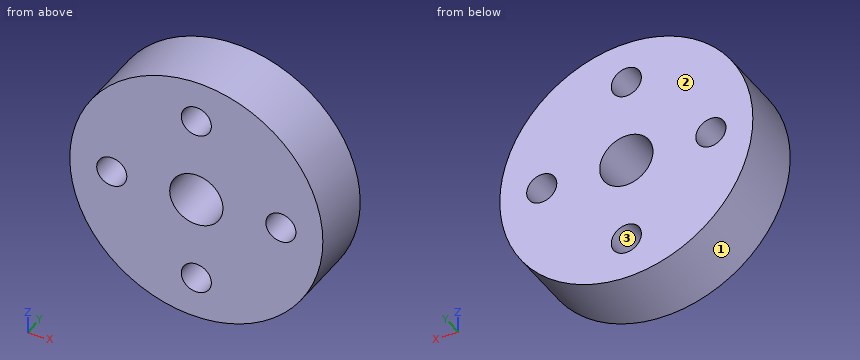
Autodesk Inventor part; units mm, degrees
ref_plane "YZ Plane" through (0, 0, 0) normal (1, 0, 0) x (0, 1, 0)
ref_plane "XZ Plane" through (0, 0, 0) normal (0, 1, 0) x (-1, 0, 0)
ref_plane "XY Plane" through (0, 0, 0) normal (0, 0, 1) x (1, 0, 0)
sketch "Sketch1" plane through (0, 0, 0) normal (0, 1, 0) x (-1, 0, 0)
  circle A0 centre (0, 0) radius 9.5
  circle A1 centre (0, 0) radius 2
  circle A2 centre (-6.35, 0) radius 1.1303
  circle A3 centre (0, -6.35) radius 1.1303
  circle A4 centre (6.35, 0) radius 1.1303
  circle A5 centre (0, 6.35) radius 1.1303
  dimension "d0" = 19
  dimension "d1" = 4
  dimension "d2" = 6.35
  dimension "d3" = 2.2606
  dimension "d6" = 360
extrude "Extrusion1" add sketch "Sketch1" along normal blind 5
properties part number "Motor_Hub_Polulu"
The listing builds one solid part. Answer for the finished solid, in the listing's coordinates (mm). Face numbers are marked on the shaded views. Coordinates: 2 decimals unless noted, no trailing zeros. Write each loop counter-clockwise with the first axis right and the second up, starting at its lowest first coordinate (ties: lowest second). Pieces come first, ordered by that corner, then holes. Notation, with made-up numbers: M 55.5,39.25 L 90.5,39.25 A27 cw 90.5,56.25 Z; hole C -34,87.25 d8. An arc over 180 degrees is marked long. Use a Markdown table: item, result. Add a question column.
1. Section C-C (z = 7) is taken. Give the vertices of the cut face in (x, y), plus the area to 3 significant figures.
2. Section B-B (z = 0) is taken. Give the vertices of the cut face in (x, y).
3. Section D-D (y = 2.95) is taken. Give the vertices of the cut face in (x, z), plus the area to 3 significant figures.
4. For a pull along X with two mould halves and no side action, classify the marked faces 1, 2 and 3 as +X half, -X half, draft (parallel to the pull), parting line (faces both ways), or undercut.
5. Given P1, Ø2, axis at x = -6.35, z = 0, coming from the +Y side; P2, Ø1, axis at x = 2, y = 1.5, coming from the -Z side; P3, Ø2, axis at y = 3.5, z = 3, coming from the -X side, each flat-ended and moving along its own axis, determine where each tip first touches the part or whether it passes through.
6. Section A-A (x = 0) is taken. Give the vertices of the cut face in (y, z), plus the area to 3 significant figures.
7. Straight lines are drawn through the part: line 1 along Z through (x, y) = (0, 3.25); line 2 along X through (y, z) = (1.7, 6); line 3 along Z through (x, y) = (-1.75, 1.8). For each, find the intervals that lie inside material, in ascending order. Write a range as [from, to].
Data:
| question | item | result |
|---|---|---|
| 1 | outline | M -6.42,0 L -0.92,0 L -0.92,5 L -6.42,5 Z; M 0.92,0 L 6.42,0 L 6.42,5 L 0.92,5 Z |
| 1 | area | 55.0 mm2 |
| 2 | outline | M -9.5,0 L -7.48,0 L -7.48,5 L -9.5,5 Z; M -5.22,0 L -2,0 L -2,5 L -5.22,5 Z; M 2,0 L 5.22,0 L 5.22,5 L 2,5 Z; M 7.48,0 L 9.5,0 L 9.5,5 L 7.48,5 Z |
| 3 | outline | C 0,0 d19; hole C -6.35,0 d2.26; hole C 0,0 d4; hole C 0,-6.35 d2.26; hole C 0,6.35 d2.26; hole C 6.35,0 d2.26 |
| 3 | area | 255 mm2 |
| 4 | face 1 | parting line |
| 4 | face 2 | draft |
| 4 | face 3 | undercut |
| 5 | P1 | passes through |
| 5 | P2 | stops at z = -9.38 |
| 5 | P3 | stops at x = -9.29 |
| 6 | outline | M 0,-9.5 L 5,-9.5 L 5,-7.48 L 0,-7.48 Z; M 0,-5.22 L 5,-5.22 L 5,-2 L 0,-2 Z; M 0,2 L 5,2 L 5,5.22 L 0,5.22 Z; M 0,7.48 L 5,7.48 L 5,9.5 L 0,9.5 Z |
| 6 | area | 52.4 mm2 |
| 7 | line 1 | z = [-9.5, -7.48], [-5.22, -2], [2, 5.22], [7.48, 9.5] |
| 7 | line 2 | x = [-7.37, -1.07], [1.07, 7.37] |
| 7 | line 3 | z = [-9.34, -0.97], [0.97, 9.34] |
